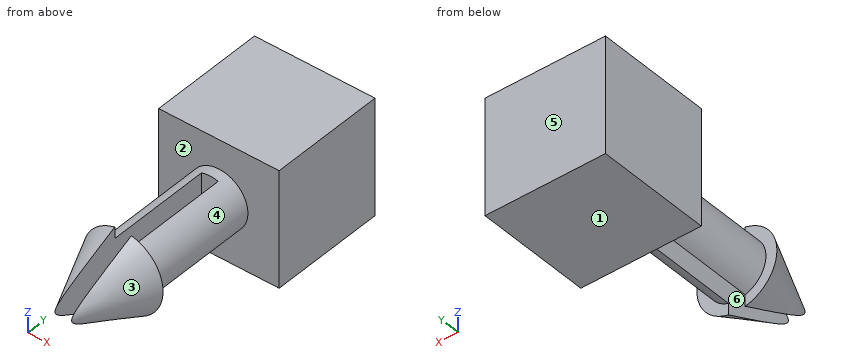
```python
from build123d import *

# Parameters (mm, degrees)
F0_W      = 13.1792449958
F0_H      = 12.7
F1_DEPTH  = 12.7
F2_R      = 3.175
F3_DEPTH  = 12.7
F7_R      = 4.375
F9_W      = 1.821417918
F9_H      = 11
F10_DEPTH = 21.5


with BuildPart() as f1:
    # F0 (on Front) → F1 (new body)
    with BuildSketch(Plane.XZ):
        Rectangle(F0_W, F0_H)
    extrude(amount=F1_DEPTH)

    # F2 (on face) → F3 (join)
    with BuildSketch(Plane.XZ.offset(12.7)):
        Circle(F2_R)
    extrude(amount=F3_DEPTH)

    # F7 (on offset) → F8 section 0
    with BuildSketch(Plane.XZ.offset(25.4), mode=Mode.PRIVATE) as f8_s0:
        Circle(F7_R)
    loft([f8_s0.sketch, Vertex(0, -35.4, 0)])

    # F9 (on offset) → F10 (cut)
    with BuildSketch(Plane.XZ.offset(35.4)):
        Rectangle(F9_W, F9_H)
    extrude(amount=-F10_DEPTH, mode=Mode.SUBTRACT)


solid = f1.part
```
Here's how the part is built. I have some questions about the finished solid (model axes, mm). Face numbers are marked on the shaded views. A direction names the side the tool comes from. Round coordinates to 2 decimals unless told otherwise and drop trailing zeros. Order: outer loops, then holes, each group sorted by start corner. A loop starts at its lowest first (then second) coordinate and runs counter-clockwise, first axis right, second up. Notation, with made-up numbers: (34.5, 67.25) -> (78.5, 67.25) arc R6 cw to (78.5, 77.25) -> close; hole circle Ø1 at (81, -1). An arc over 180 degrees is marked (long way). Use a Markdown table: item, result. Add a question column.
(1) Suppose I cut it at D-D, the plane z = 3.75. Count the separate pieces of the cut face and the enclosed holes in it, and give its area (3 significant figures).
(2) Suppose I cut it at B-B, the plane x = 0. Please give me the cut outline in (y, z) (3 decimals).
(3) For pin 1 Ø1.5 at (x, z) = (0, 1.5) entering from -Y; pin 2 Ø4.5 at (y, z) = (-25, -0.5) entering from -X (3 decimals); pin 3 Ø4 at (x, y) = (1.5, -17) entering from +Z, each with a flat end and sliding along its axis, tell me the tip position at first contact or that it passes through.
(4) Suppose I cut it at C-C, the plane y = -29.5. Please give me the cut outline in (x, z).
(5) I need wall thicknesses on line 1 along Y through (x, z) = (-4, 3); line 2 along Y through (x, z) = (-2, 3.5); line 3 along X through (y, z) = (-26, 2.5). Which ranges of each line are inside material? Lowest first, please.
(6) If we mould it in two halves opening along Y, with no side actions, what happens to the marked faces 1, 2 and 3? For each: released by +Y, released by -Y, zero draft, split by the parting line, or undercut.
(7) For the marked faces 4, 5 and 6, which set-ups out of +Z, -Z, +X, -X, +Y, -Y let a thin tool reach every point of the face, with its end or its side?
(8) Suppose I cut it at A-A, the plane z = 0. Please give me the cut outline in (x, y) (3 decimals).
Verdict:
| question | item | result |
|---|---|---|
| 1 | separate pieces | 3 |
| 1 | enclosed holes | 0 |
| 1 | area | 169 mm2 |
| 2 | outline | (-13.9, -3.175) -> (-12.7, -3.175) -> (-12.7, -6.35) -> (0, -6.35) -> (0, 6.35) -> (-12.7, 6.35) -> (-12.7, 3.175) -> (-13.9, 3.175) -> close |
| 3 | pin 1 | y = -13.9 |
| 3 | pin 2 | x = -4.375 |
| 3 | pin 3 | z = 3.04 |
| 4 | outline | (-0.91, -2.42) -> (-0.91, 2.42) arc R2.58 ccw to start; (0.91, -2.42) arc R2.58 ccw to (0.91, 2.42) -> close |
| 5 | line 1 | -12.7 to 0 |
| 5 | line 2 | -26.19 to -25.4, -12.7 to 0 |
| 5 | line 3 | -3.27 to -0.91, 0.91 to 3.27 |
| 6 | face 1 | zero draft |
| 6 | face 2 | undercut |
| 6 | face 3 | released by -Y |
| 7 | face 4 | none |
| 7 | face 5 | +Z, -Z, +X, -X, +Y |
| 7 | face 6 | +Z, -Z, -Y |
| 8 | outline | (-6.59, -12.7) -> (-3.175, -12.7) -> (-3.175, -25.4) -> (-4.375, -25.4) -> (-0.911, -33.318) -> (-0.911, -13.9) -> (0.911, -13.9) -> (0.911, -33.318) -> (4.375, -25.4) -> (3.175, -25.4) -> (3.175, -12.7) -> (6.59, -12.7) -> (6.59, 0) -> (-6.59, 0) -> close |
